The listing builds one solid part. Answer for the finished solid, in the listing's coordinates (mm). A direction names the side the tool comes from. Coordinates: 2 decimals unless noted, no trailing zeros. Order: outer loops, then holes, each group sorted by start corner. A loop starts at its lowest first (then second) coordinate and runs counter-clockwise, first axis right, second up.
```python
from build123d import *

# Parameters (mm, degrees)
BOSS_EXTRUDE1_DEPTH     = 23
CUT_EXTRUDE2_DEPTH      = 23
CUT_EXTRUDE2_DEPTH_BACK = 10
SKETCH4_W               = 3.5
SKETCH4_H               = 21
SKETCH5_W               = 45
SKETCH5_H               = 7.5
CUT_EXTRUDE3_DEPTH      = 26
SKETCH7_R               = 1.45
CUT_EXTRUDE4_DEPTH      = 50
SKETCH8_W               = 13
SKETCH8_H               = 15.5
BOSS_EXTRUDE2_DEPTH     = 2.5
SKETCH9_R               = 1.45
CUT_EXTRUDE5_DEPTH      = 10


with BuildPart() as part:
    # Sketch1 → Boss-Extrude1 (new body)
    with BuildSketch(Plane.XY):
        with BuildLine():
            Line((0, 3), (0, 17))
            ThreePointArc((0, 17), (1.464466094, 20.535533906), (5, 22))
            Line((5, 22), (22, 22))
            ThreePointArc((22, 22), (25.535533906, 20.535533906), (27, 17))
            Line((27, 17), (27, 3))
            ThreePointArc((27, 3), (27.878679656, 0.878679656), (30, 0))
            Line((30, 0), (36, 0))
            Line((36, 0), (36, -4))
            Line((36, -4), (23, -4))
            Line((23, -4), (23, 18))
            Line((23, 18), (4, 18))
            Line((4, 18), (4, -4))
            Line((4, -4), (-9, -4))
            Line((-9, -4), (-9, 0))
            Line((-9, 0), (-3, 0))
            ThreePointArc((-3, 0), (-0.878679656, 0.878679656), (0, 3))
        make_face()
    extrude(amount=BOSS_EXTRUDE1_DEPTH)

    # Sketch4 → Cut-Extrude2 (cut, two sides: drawn at the far end of the back side and taken through both)
    with BuildSketch(Plane.ZY.offset(-CUT_EXTRUDE2_DEPTH_BACK)):
        with Locations((5.75, 6.5)):
            Rectangle(SKETCH4_W, SKETCH4_H)
    extrude(amount=CUT_EXTRUDE2_DEPTH + CUT_EXTRUDE2_DEPTH_BACK, mode=Mode.SUBTRACT)

    # Sketch5 → Cut-Extrude3 (cut)
    with BuildSketch(Plane(origin=(0, 22, 0), x_dir=(1, 0, 0), z_dir=(0, 1, 0))):
        with Locations((13.5, -3.75)):
            Rectangle(SKETCH5_W, SKETCH5_H)
    extrude(amount=-CUT_EXTRUDE3_DEPTH, mode=Mode.SUBTRACT)

    # Sketch7 → Cut-Extrude4 (cut)
    with BuildSketch(Plane(origin=(0, 0, 0), x_dir=(1, 0, 0), z_dir=(0, 1, 0))):
        with Locations(Location((-6, -15.25, 0), (0, 0, 270))):
            Circle(SKETCH7_R)
        with Locations(Location((33, -15.25, 0), (0, 0, 180))):
            Circle(SKETCH7_R)
    extrude(amount=-CUT_EXTRUDE4_DEPTH, mode=Mode.SUBTRACT)

    # Sketch8 → Boss-Extrude2 (add)
    with BuildSketch(Plane.XZ.offset(4)):
        with Locations((29.5, 15.25)):
            Rectangle(SKETCH8_W, SKETCH8_H)
        with Locations((-2.5, 15.25)):
            Rectangle(SKETCH8_W, SKETCH8_H)
    extrude(amount=BOSS_EXTRUDE2_DEPTH)

    # Sketch9 → Cut-Extrude5 (cut)
    with BuildSketch(Plane(origin=(0, -4, 0), x_dir=(1, 0, 0), z_dir=(0, 1, 0))):
        with Locations((33, -15.25)):
            Circle(SKETCH9_R)
        with Locations(Location((-6, -15.25, 0), (0, 0, 270))):
            Circle(SKETCH9_R)
    extrude(amount=-CUT_EXTRUDE5_DEPTH, mode=Mode.SUBTRACT)


solid = part.part
```
1) A cutting plane is placed at B-B, the plane z = 15.25. Write down the section's boundary in (x, y).
2) The mould has two halves that part along X. Classify faces 5 (the flat face through (36, -3, 15)), 6 (the flat face through (-9, -3, 15)), 7 (the flat face through (14, 18, 15)): released by +X, released by -X, zero draft, split by the parting line, or undercut.
3) A cutting plane is placed at D-D, the plane z = 22.25. Write down the section's boundary in (x, y).
4) Each of these flat-tipped pins is pushed along its axis until it touches: P1, Ø8, axis at x = 17.5, z = 15.5, coming from the -Y side; P2, Ø3.5, axis at x = -6, z = 15.25, coming from the +Y side; P3, Ø4.5, axis at y = 3, z = 14, coming from the +X side. Where does it stop, or does it pass through?
5) A cutting plane is placed at C-C, the plane y = 15. Write down the section's boundary in (x, z), plus the area to 3 significant figures.
6) For faces 1 (the flat face through (33, 0, 17)), 2 (the flat face through (0, 10, 15)), 3 (the flat face through (4, 6, 15)), 4 (the flat face through (13, 22, 15)), determine the directions among +Z, -Z, +X, -X, +Y, -Y from which every point of the face is accessible in a straight line to the end or side of a thin tool.
7) A cutting plane is placed at A-A, the plane x = -6. Write down the section's boundary in (y, z).
8) Straight lines are drawn through the part: probe 1 along X at (y, z) = (-0.95, 15.25); probe 2 along X at (y, z) = (6.5, 10); probe 3 along Z at (x, y) = (33, -5.15). For each, find the intervals that lie inside material, in ascending order.
Working result:
1. outline: (-9, -6.5) - (-7.45, -6.5) - (-7.45, 0) - (-9, 0) - close; (-4.55, -6.5) - (4, -6.5) - (4, 18) - (23, 18) - (23, -6.5) - (31.55, -6.5) - (31.55, 0) - (30, 0) arc R3 cw to (27, 3) - (27, 17) arc R5 ccw to (22, 22) - (5, 22) arc R5 ccw to (0, 17) - (0, 3) arc R3 cw to (-3, 0) - (-4.55, 0) - close; (34.45, -6.5) - (36, -6.5) - (36, 0) - (34.45, 0) - close
2. face 5: released by +X
2. face 6: released by -X
2. face 7: undercut
3. outline: (-9, -6.5) - (4, -6.5) - (4, 18) - (23, 18) - (23, -6.5) - (36, -6.5) - (36, 0) - (30, 0) arc R3 cw to (27, 3) - (27, 17) arc R5 ccw to (22, 22) - (5, 22) arc R5 ccw to (0, 17) - (0, 3) arc R3 cw to (-3, 0) - (-9, 0) - close
4. P1: stops at y = 18
4. P2: stops at y = 0
4. P3: stops at x = 28.02
5. outline: (0, 7.5) - (4, 7.5) - (4, 23) - (0, 23) - close; (23, 7.5) - (27, 7.5) - (27, 23) - (23, 23) - close
5. area: 124 mm2
6. face 1: +Z, -Z, +X, +Y
6. face 2: +Z, -Z, -X, +Y
6. face 3: +Z, -Z, -Y
6. face 4: +Z, -Z, +X, -X, +Y
7. outline: (-6.5, 7.5) - (0, 7.5) - (0, 13.8) - (-6.5, 13.8) - close; (-6.5, 16.7) - (0, 16.7) - (0, 23) - (-6.5, 23) - close
8. probe 1: x = -9 to -7.45, -4.55 to 4, 23 to 31.55, 34.45 to 36
8. probe 2: x = 0 to 4, 23 to 27
8. probe 3: z = 7.5 to 13.8, 16.7 to 23
